Geometry check sheet. Reference: the model listing, model coordinates, mm. Face numbers are marked on the shaded views. A direction names the side the tool comes from. Give positions to 0.01 mm unless a question says otherwise; leave off trailing zeros. Write each loop counter-clockwise with the first axis right and the second up, starting at its lowest first coordinate (ties: lowest second). Pieces come first, ordered by that corner, then holes. Notation, with made-up numbers: (1, 80) - (57, 80) arc R14 cw to (57, 90) - close; hole circle Ø3 at (64.5, 52.5). An arc over 180 degrees is marked (long way). Write item = value, one per line. Start each with the question number.
(1) Depth check by flat-ended pin: pin 1 Ø1.5 at (y, z) = (-105.5, 46.5) entering from -X; pin 2 Ø12 at (y, z) = (-79, -13.5) entering from -X; pin 3 Ø6 at (x, y) = (-14.5, 2) entering from +Z; pin 4 Ø5 at (x, z) = (12, 2.5) entering from +Y. Enter the tip coordinate at first touch or a pass-through.
(2) Thickness scan on L1, parallel to Y at x = -31, z = -43; L2, parallel to X at y = 0.5, z = -65. Record the ranges inside material, lowest first.
(3) Section check D-D, the plane z = -20. Enter the section's corners in (x, y).
(4) Access from +Z, -Z, +X, -X, +Y, -Y to the whole of each face (thin tool, end or side, straight path). Record for the marked faces 1, 2, 3 and 4.
```python
from build123d import *

# Parameters (mm, degrees)
F1_DEPTH = 80
F3_DEPTH = 130
F5_DEPTH = 130
F7_DEPTH = 5.734064
F9_DEPTH = 5.734064


with BuildPart() as f1:
    # F0 (on Top) → F1 (new body)
    with BuildSketch(Plane.XY):
        Polygon((-130, 7), (-130, 0), (0, 0), (0, -130), (7, -130), (7, 7), align=None)
    extrude(amount=-F1_DEPTH)

    # F2 (on face) → F3 (join)
    with BuildSketch(Plane.XZ.offset(130)):
        Polygon((57.357644, 81.915204), (0, 0), (7, 0), (64.357644, 81.915204), align=None)
    extrude(amount=-F3_DEPTH)

    # F4 (on face) → F5 (join)
    with BuildSketch(Plane(origin=(-130, 0, 0), x_dir=(0, -1, 0), z_dir=(-1, 0, 0))):
        Polygon((-7, 0), (0, 0), (-57.357644, 81.915204), (-64.357644, 81.915204), align=None)
    extrude(amount=-F5_DEPTH)

    # F6 (on face) → F7 (join, through all)
    with BuildSketch(Plane(origin=(4.697071, 0, -3.288924), x_dir=(0, 1, 0), z_dir=(0.819152, 0, -0.573576))):
        Polygon((60.783785, 104.015035), (0, 104.015035), (0, 4.015035), align=None)
    extrude(amount=-F7_DEPTH)

    # F8 (on face) → F9 (join, through all)
    with BuildSketch(Plane(origin=(0, 4.697071, -3.288924), x_dir=(-1, 0, 0), z_dir=(0, 0.819152, -0.573576))):
        Polygon((0, 4.015035), (0, 104.015035), (-56.736283, 104.015035), align=None)
    extrude(amount=-F9_DEPTH)


solid = f1.part
```
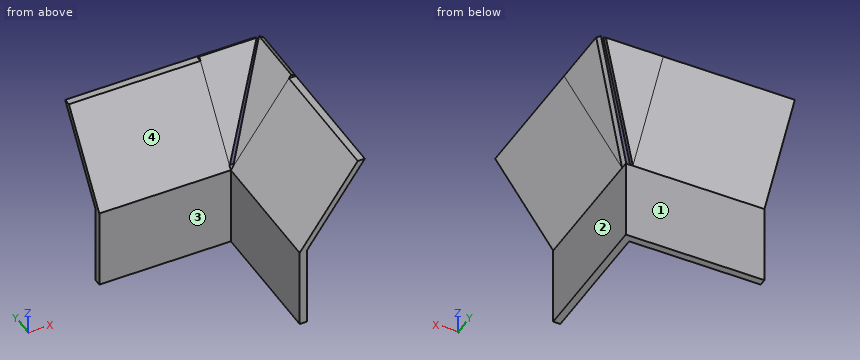
Model answer:
q1.pin_1 = 32.03
q1.pin_2 = 0
q1.pin_3 = 7.14
q1.pin_4 = through
q2.L1 = 0 to 7
q2.L2 = -130 to 7
q3.outline = (-130, 0) - (0, 0) - (0, -130) - (7, -130) - (7, 7) - (-130, 7) - close
q4.face_1 = -Z, +X, -X, +Y
q4.face_2 = -Z, +X, +Y, -Y
q4.face_3 = +Z, -Z, -X, -Y
q4.face_4 = +Z, -X, -Y
